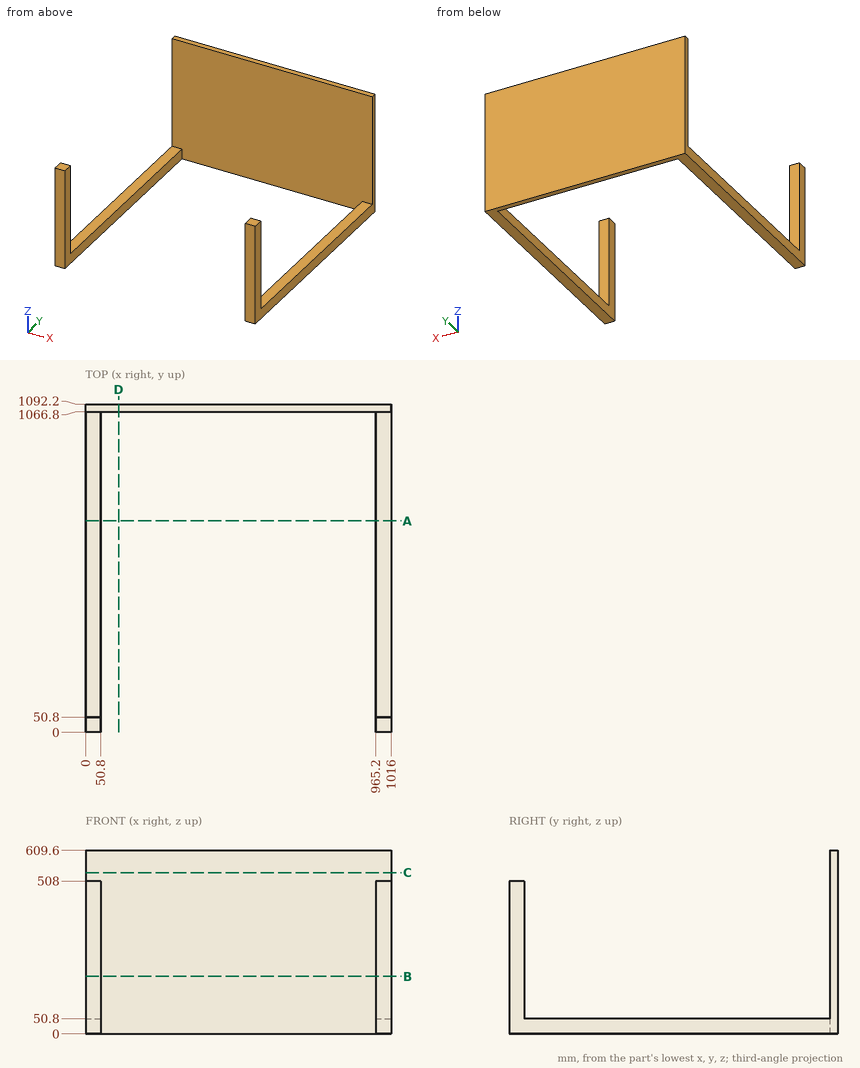
Here's the drawing with two shaded views (mm, measured from the low corner). I have some questions. Give positions to 0.01 mm unless a question says otherwise; leave off trailing zeros. Loops run counter-clockwise (first coordinate to the right, second up) from the corner with the lowest first, then second, coordinate; pieces in that order, holes last. Notation, with made-up numbers: M 32,57.5 L 82,57.5 A18 cw 82,72.5 Z; hole C 5.25,-25.75 d8. An arc over 180 degrees is marked long. Use one line per item in the form item = value. Start each with the question number.
Q1. I need wall thicknesses on line 1 along X through (y, z) = (553.5, 49.5); line 2 along Y through (x, z) = (688, 265). Which ranges of each line are inside material? Lowest first, please.
Q2. If we section it at A-A (y = 703.5): Write out the boundary of the cut face in (x, z), then the cut area to 3 significant figures.
Q3. If we section it at C-C (z = 536): Write out the boundary of the cut face in (x, y), then the cut area to 3 significant figures.
Q4. If we section it at D-D (x = 110.5): Write out the boundary of the cut face in (y, z).
Q5. If we section it at B-B (z = 191): Write out the boundary of the cut face in (x, y).
Q6. Will these pins go through, and if not, where does the flat tip stop? pin 1 Ø6 at (x, z) = (794, 281) entering from -Y; pin 2 Ø15 at (x, y) = (14, 28) entering from +Z; pin 3 Ø15 at (x, y) = (29, 751.5) entering from +Z.
Taken from the geometry:
q1.line_1 = 0 to 50.8, 965.2 to 1016
q1.line_2 = 1066.8 to 1092.2
q2.outline = M 0,0 L 50.8,0 L 50.8,50.8 L 0,50.8 Z; M 965.2,0 L 1016,0 L 1016,50.8 L 965.2,50.8 Z
q2.area = 5,160 mm^2
q3.outline = M 0,1066.8 L 1016,1066.8 L 1016,1092.2 L 0,1092.2 Z
q3.area = 25,800 mm^2
q4.outline = M 1066.8,0 L 1092.2,0 L 1092.2,609.6 L 1066.8,609.6 Z
q5.outline = M 0,0 L 50.8,0 L 50.8,50.8 L 0,50.8 Z; M 0,1066.8 L 1016,1066.8 L 1016,1092.2 L 0,1092.2 Z; M 965.2,0 L 1016,0 L 1016,50.8 L 965.2,50.8 Z
q6.pin_1 = 1066.8
q6.pin_2 = 508
q6.pin_3 = 50.8
